Read the model definition and answer for the solid it produces. Units are mm, in the model's axes. Face numbers are marked on the shaded views. A direction names the side the tool comes from. Coordinates: 2 decimals unless noted, no trailing zeros. Write each loop counter-clockwise with the first axis right and the second up, starting at its lowest first coordinate (ties: lowest second). Pieces come first, ordered by that corner, then holes. Notation, with made-up numbers: (56, 35.25) - (71, 35.25) arc R22 ccw to (71, 63.25) - close; hole circle Ø9 at (-5.5, 7). An arc over 180 degrees is marked (long way). Return JSON: item names as keys, results as strings.
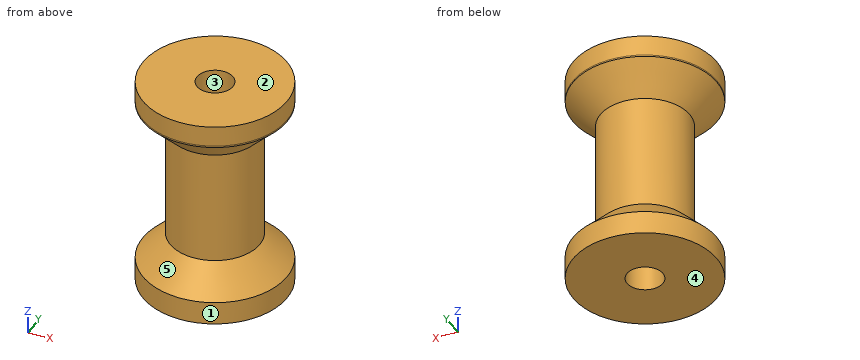
```python
from build123d import *

# Parameters (mm, degrees)
F0_R         = 12.7
F1_DEPTH     = 38.1
F2_W         = 10.2602215484
F2_H         = 30.5833565071
F4_R         = 3.175
F5_DEPTH     = 50.8
F6_S5_R      = 12.7
F6_T6_DEPTH  = 20
F6_S11_R     = 12.7
F6_T12_DEPTH = 20


# Not quite as in the source:
# - a fillet or chamfer that OpenCascade refuses, or shapes differently, is made with other operations: its cross-section is extruded or revolved along the edge and cut away or added


with BuildPart() as f1:
    # F0 (on Top) → F1 (new body)
    with BuildSketch(Plane.XY):
        Circle(F0_R)
    extrude(amount=F1_DEPTH)

    # F2 (on Right) → F3 (revolve, cut)
    with BuildSketch(Plane.YZ):
        with Locations((-13.0225899629, 19.1392614506)):
            Rectangle(F2_W, F2_H)
    revolve(axis=Axis((0, 0, 18.941948656), (0, 0, -1)), mode=Mode.SUBTRACT)

    # F4 (on face) → F5 (cut)
    with BuildSketch(Plane(origin=(0, 0, 0), x_dir=(1, 0, 0), z_dir=(0, 0, -1))):
        Circle(F4_R)
    extrude(amount=-F5_DEPTH, mode=Mode.SUBTRACT)

    # F6: chamfer of 5.08 on 2 edges, made by hand


with BuildPart() as f6_tool2:
    # F6_s3 → F6_t4 (revolve)
    with BuildSketch(Plane.YZ):
        Polygon((-12.9724791887, 3.8475831971), (-7.8924791887, 8.9275831971), (-7.8924791887, 3.8475831971), align=None)
    revolve(axis=Axis((0, 0, 3.8475831971), (0, 0, -1)))

    # F6_s5 → F6_t6 (intersect, symmetric)
    with BuildSketch(Plane.XY.offset(6.4)):
        Circle(F6_S5_R)
    extrude(amount=F6_T6_DEPTH, both=True, mode=Mode.INTERSECT)


with BuildPart() as f1_1:
    add(f1.part)

    # F6_t1: union F6_tool2
    add(f6_tool2.part)


with BuildPart() as f6_tool8:
    # F6_s9 → F6_t10 (revolve)
    with BuildSketch(Plane.YZ):
        Polygon((-7.8924791887, 29.3509397042), (-12.9724791887, 34.4309397042), (-7.8924791887, 34.4309397042), align=None)
    revolve(axis=Axis((0, 0, 34.4309397042), (0, 0, -1)))

    # F6_s11 → F6_t12 (intersect, symmetric)
    with BuildSketch(Plane.XY.offset(31.9)):
        Circle(F6_S11_R)
    extrude(amount=F6_T12_DEPTH, both=True, mode=Mode.INTERSECT)


with BuildPart() as f1_2:
    add(f1_1.part)

    # F6_t7: union F6_tool8
    add(f6_tool8.part)


solid = f1_2.part
```
(1) Straight lines are drawn through the part: line 1 (Y direction, x = 0, z = 17.5) (3 decimals); line 2 (Z direction, x = 2.25, y = 8.5). For each, find the intervals that lie inside material, in ascending order. Write a range as from..to.
Answer:
{"line 1": "-7.892..-3.175, 3.175..7.892", "line 2": "0..8.03, 30.25..38.1"}
(2) Which of the six approach directions +Z, -Z, +X, -X, +Y, -Y give full straight-line access (tool end or side, diameter ignored) to the marked faces 4 and 5?
Answer:
{"face 4": "-Z, +X, -X, +Y, -Y", "face 5": "none"}
(3) Determine the mould class of the marked faces 1, 2 and 3 for opening direction X: +X half, -X half, draft (parallel to the pull), parting line (faces both ways), or undercut.
Answer:
{"face 1": "parting line", "face 2": "draft", "face 3": "undercut"}
(4) A cutting plane is placed at C-C (z = 3). Determine the outline of the cut face in (x, y) (3 decimals), and give its area (3 significant figures).
Answer:
{"outline": "circle Ø25.4 at (0, 0); hole circle Ø6.35 at (0, 0)", "area": "475 mm²"}
(5) A cutting plane is placed at A-A (x = 0). Determine the outline of the cut face in (y, z) (3 decimals), and give its area (3 significant figures).
Answer:
{"outline": "(-12.7, 0) - (-3.175, 0) - (-3.175, 38.1) - (-12.7, 38.1) - (-12.7, 34.158) - (-7.892, 29.351) - (-7.892, 8.928) - (-12.7, 4.12) - close; (3.175, 0) - (12.7, 0) - (12.7, 4.12) - (7.892, 8.928) - (7.892, 29.351) - (12.7, 34.158) - (12.7, 38.1) - (3.175, 38.1) - close", "area": "483 mm²"}
(6) A cutting plane is placed at D-D (z = 21). Determine the outline of the cut face in (x, y) (3 decimals), and give its area (3 significant figures).
Answer:
{"outline": "circle Ø15.785 at (0, 0); hole circle Ø6.35 at (0, 0)", "area": "164 mm²"}
(7) Flat-ended cylindrical pins translate along their axes: P1, Ø4, axis at x = 1, z = 16, coming from the +Y side; P2, Ø12, axis at x = 6, z = 20.5, coming from the -Y side; P3, Ø5, axis at x = 6, z = 11, coming from the -Y side; P4, Ø5.5, axis at x = 0, y = 0, coming from the +Z side. Find the tip coordinate at first contact, or state that the pin passes through.
Answer:
{"P1": "y = 7.89", "P2": "y = -7.89", "P3": "y = -7.07", "P4": "through"}
